Verification items for the finished model (mm, model axes). Face numbers are marked on the shaded views. A direction names the side the tool comes from. Coordinates: 2 decimals unless noted, no trailing zeros. Order: outer loops, then holes, each group sorted by start corner. A loop starts at its lowest first (then second) coordinate and runs counter-clockwise, first axis right, second up. Notation, with made-up numbers: M -9,11.5 L 38,11.5 A25 ccw 38,26.5 Z; hole C 15.25,52.25 d9. An arc over 180 degrees is marked long. Return JSON: item names as keys, results as strings.
```python
from build123d import *

# Parameters (mm, degrees)
SKETCH1_W                                            = 318
SKETCH1_H                                            = 160
BOSS_EXTRUDE1_DEPTH                                  = 25
SKETCH2_R                                            = 28.5
CUT_EXTRUDE1_DEPTH                                   = 180.738699228
CUT_EXTRUDE2_DEPTH                                   = 180.738699228
CUT_EXTRUDE2_DEPTH_BACK                              = 180.738699228
SKETCH4_R                                            = 9.55
CHAMFER1_SIZE                                        = 0.5
FILLET1_R                                            = 20
M8_CLEARANCE_HOLE1_D                                 = 9
M6X1_0_TAPPED_HOLE1_D                                = 5
SKETCH13_R                                           = 13.411040831
SKETCH13_R_2                                         = 14.724493856
BOSS_EXTRUDE3_DEPTH                                  = 8
CSK_FOR_5_16_FLAT_HEAD_SOCKET_CAP_SCREW1_D           = 8.4328
CSK_FOR_5_16_FLAT_HEAD_SOCKET_CAP_SCREW1_CSINK_D     = 18.4009792
CSK_FOR_5_16_FLAT_HEAD_SOCKET_CAP_SCREW1_CSINK_ANGLE = 82
BOSS_EXTRUDE4_DEPTH                                  = 6
CUT_EXTRUDE3_DEPTH                                   = 186.067555233
M6X1_0_TAPPED_HOLE2_D                                = 5
M6X1_0_TAPPED_HOLE2_DEPTH                            = 15
M6X1_0_TAPPED_HOLE2_TIP                              = 1.502151548
MIRROR2_COPY_1_DEPTH                                 = 186.067555233
CHAMFER4_SIZE                                        = 1


with BuildPart() as part:
    # Sketch1 → Boss-Extrude1 (new body)
    with BuildSketch(Plane(origin=(0, 0, 0), x_dir=(1, 0, 0), z_dir=(0, 1, 0))):
        Rectangle(SKETCH1_W, SKETCH1_H)
    extrude(amount=BOSS_EXTRUDE1_DEPTH)

    # Sketch2 → Cut-Extrude1 (cut, through all)
    with BuildSketch(Plane(origin=(0, 25, 0), x_dir=(1, 0, 0), z_dir=(0, 1, 0))):
        with Locations(Location((-114, 0, 0), (0, 0, 270))):
            Circle(SKETCH2_R)
        with Locations(Location((114, 0, 0), (0, 0, 270))):
            Circle(SKETCH2_R)
    extrude(amount=-CUT_EXTRUDE1_DEPTH, mode=Mode.SUBTRACT)

    # Sketch4 → Cut-Extrude2 (cut, two sides: drawn at the far end of the back side and taken through both)
    with BuildSketch(Plane(origin=(0, 25, 0), x_dir=(1, 0, 0), z_dir=(0, 1, 0)).offset(-CUT_EXTRUDE2_DEPTH_BACK)):
        with Locations(Location((-60, 0, 0), (0, 0, 270))):
            Circle(SKETCH4_R)
        with Locations(Location((60, 0, 0), (0, 0, 270))):
            Circle(SKETCH4_R)
    extrude(amount=CUT_EXTRUDE2_DEPTH + CUT_EXTRUDE2_DEPTH_BACK, mode=Mode.SUBTRACT)

    # Chamfer1
    chamfer1_edges = [part.edges().sort_by_distance(p)[0] for p in [
        (-114, 0, -28.5),
        (-114, 25, -28.5),
        (114, 0, -28.5),
        (114, 25, -28.5),
        (-60, 0, -9.55),
        (-60, 25, -9.55),
        (60, 0, -9.55),
        (60, 25, -9.55),
    ]]
    chamfer(chamfer1_edges, length=CHAMFER1_SIZE)

    # Fillet1
    fillet1_edges = [part.edges().sort_by_distance(p)[0] for p in [
        (159, 12.5, 80),
        (-159, 12.5, 80),
        (-159, 12.5, -80),
        (159, 12.5, -80),
    ]]
    fillet(fillet1_edges, radius=FILLET1_R)

    # M8 Clearance Hole1 (through all)
    with Locations(Plane.XZ):
        with Locations((-139, -60), (-139, 60), (139, -60), (139, 60)):
            Hole(M8_CLEARANCE_HOLE1_D / 2)

    # M6x1.0 Tapped Hole1 (through all)
    with Locations(Plane(origin=(0, 0, 0), x_dir=(-1, 0, 0), z_dir=(0, -1, 0))):
        with Locations((138.765, -24.765), (89.235, -24.765), (89.235, 24.765), (138.765, 24.765), (-89.235, -24.765), (-138.765, -24.765), (-89.235, 24.765), (-138.765, 24.765)):
            Hole(M6X1_0_TAPPED_HOLE1_D / 2)

    # Sketch13 → Boss-Extrude3 (add)
    with BuildSketch(Plane(origin=(0, 25, 0), x_dir=(1, 0, 0), z_dir=(0, 1, 0))):
        with Locations((60, 0)):
            Circle(SKETCH13_R)
        with Locations((-60, 0)):
            Circle(SKETCH13_R_2)
    extrude(amount=-BOSS_EXTRUDE3_DEPTH)

    # CSK for 5/16 Flat Head Socket Cap Screw1 (through all)
    with Locations(Plane(origin=(0, 25, 0), x_dir=(1, 0, 0), z_dir=(0, 1, 0))):
        with Locations((60, 0), (-60, 0)):
            CounterSinkHole(CSK_FOR_5_16_FLAT_HEAD_SOCKET_CAP_SCREW1_D / 2, CSK_FOR_5_16_FLAT_HEAD_SOCKET_CAP_SCREW1_CSINK_D / 2, counter_sink_angle=CSK_FOR_5_16_FLAT_HEAD_SOCKET_CAP_SCREW1_CSINK_ANGLE)

    # Sketch16 → Boss-Extrude4 (add)
    with BuildSketch(Plane.XZ.offset(-25)):
        with BuildLine():
            Line((163, -60), (163, 60))
            ThreePointArc((163, 60), (155.970562748, 76.970562748), (139, 84))
            Line((139, 84), (-139, 84))
            ThreePointArc((-139, 84), (-155.970562748, 76.970562748), (-163, 60))
            Line((-163, 60), (-163, -60))
            ThreePointArc((-163, -60), (-155.970562748, -76.970562748), (-139, -84))
            Line((-139, -84), (139, -84))
            ThreePointArc((139, -84), (155.970562748, -76.970562748), (163, -60))
        make_face()
        with BuildLine():
            Line((159, 60), (159, -60))
            ThreePointArc((159, -60), (153.142135624, -74.142135624), (139, -80))
            Line((139, -80), (-139, -80))
            ThreePointArc((-139, -80), (-153.142135624, -74.142135624), (-159, -60))
            Line((-159, -60), (-159, 60))
            ThreePointArc((-159, 60), (-153.142135624, 74.142135624), (-139, 80))
            Line((-139, 80), (139, 80))
            ThreePointArc((139, 80), (153.142135624, 74.142135624), (159, 60))
        make_face(mode=Mode.SUBTRACT)
    extrude(amount=BOSS_EXTRUDE4_DEPTH)

    # Sketch17 → Cut-Extrude3 (cut, through all)
    with BuildSketch(Plane.XZ):
        with BuildLine():
            Line((-60, -21.237304048), (-30, -21.237304048))
            ThreePointArc((-30, -21.237304048), (-16.218066161, -35.019237886), (-30, -48.801171725))
            Line((-30, -48.801171725), (-60, -48.801171725))
            ThreePointArc((-60, -48.801171725), (-73.781933839, -35.019237886), (-60, -21.237304048))
        make_face()
    cut_extrude3 = extrude(amount=-CUT_EXTRUDE3_DEPTH, mode=Mode.SUBTRACT)

    # M6x1.0 Tapped Hole2
    with Locations(Plane(origin=(0, 0, 0), x_dir=(-1, 0, 0), z_dir=(0, -1, 0))):
        with Locations((-75, 70), (-45, 70), (-105, 70), (-15, 70), (15, 70), (45, 70), (75, 70), (105, 70), (-105, -70), (-75, -70), (-45, -70), (-15, -70), (15, -70), (45, -70), (75, -70), (105, -70)):
            Hole(M6X1_0_TAPPED_HOLE2_D / 2, depth=M6X1_0_TAPPED_HOLE2_DEPTH)
            with Locations((0, 0, -(M6X1_0_TAPPED_HOLE2_DEPTH + M6X1_0_TAPPED_HOLE2_TIP / 2))):  # 118° drill point
                Cone(0, M6X1_0_TAPPED_HOLE2_D / 2, M6X1_0_TAPPED_HOLE2_TIP, mode=Mode.SUBTRACT)

    # Mirror1: Cut-Extrude3 across plane
    add(cut_extrude3.mirror(Plane(origin=(0, 0, 0), x_dir=(0, 0, 1), z_dir=(1, 0, 0))), mode=Mode.SUBTRACT)

    # Mirror2: Cut-Extrude3 across plane
    add(cut_extrude3.mirror(Plane.XY), mode=Mode.SUBTRACT)

    # Mirror2 copy 1 sketch → Mirror2 copy 1 (cut, through all)
    with BuildSketch(Plane(origin=(0, 0, 0), x_dir=(-1, 0, 0), z_dir=(0, -1, 0))):
        with BuildLine():
            Line((-60, -21.237304048), (-30, -21.237304048))
            ThreePointArc((-30, -21.237304048), (-16.218066161, -35.019237886), (-30, -48.801171725))
            Line((-30, -48.801171725), (-60, -48.801171725))
            ThreePointArc((-60, -48.801171725), (-73.781933839, -35.019237886), (-60, -21.237304048))
        make_face()
    extrude(amount=-MIRROR2_COPY_1_DEPTH, mode=Mode.SUBTRACT)

    # Chamfer4
    chamfer4_edges = [part.edges().sort_by_distance(p)[0] for p in [
        (-134.5, 0, 60),
        (-134.5, 25, 60),
        (-134.5, 0, -60),
        (-134.5, 25, -60),
        (155.970562748, 19, -76.970562748),
        (163, 19, 0),
        (155.970562748, 19, 76.970562748),
        (0, 19, 84),
        (-155.970562748, 19, 76.970562748),
        (-163, 19, 0),
        (-155.970562748, 19, -76.970562748),
        (0, 19, -84),
        (155.970562748, 25, -76.970562748),
        (163, 25, 0),
        (155.970562748, 25, 76.970562748),
        (0, 25, 84),
        (-155.970562748, 25, 76.970562748),
        (-163, 25, 0),
        (-155.970562748, 25, -76.970562748),
        (0, 25, -84),
        (-73.781933839, 25, -35.019237886),
        (-45, 25, -21.237304048),
        (-16.218066161, 25, -35.019237886),
        (-45, 25, -48.801171725),
        (-73.781933839, 0, -35.019237886),
        (-45, 0, -48.801171725),
        (-16.218066161, 0, -35.019237886),
        (-45, 0, -21.237304048),
        (73.781933839, 0, -35.019237886),
        (45, 0, -48.801171725),
        (16.218066161, 0, -35.019237886),
        (45, 0, -21.237304048),
        (73.781933839, 25, -35.019237886),
        (45, 25, -48.801171725),
        (16.218066161, 25, -35.019237886),
        (45, 25, -21.237304048),
        (73.781933839, 25, 35.019237886),
        (45, 25, 21.237304048),
        (16.218066161, 25, 35.019237886),
        (45, 25, 48.801171725),
        (73.781933839, 0, 35.019237886),
        (45, 0, 48.801171725),
        (16.218066161, 0, 35.019237886),
        (45, 0, 21.237304048),
        (-73.781933839, 0, 35.019237886),
        (-45, 0, 48.801171725),
        (-16.218066161, 0, 35.019237886),
        (-45, 0, 21.237304048),
        (-73.781933839, 25, 35.019237886),
        (-45, 25, 48.801171725),
        (-16.218066161, 25, 35.019237886),
        (-45, 25, 21.237304048),
        (159, 0, 0),
        (0, 0, 80),
        (-159, 0, 0),
        (0, 0, -80),
        (-153.142135624, 0, 74.142135624),
        (-153.142135624, 0, -74.142135624),
        (153.142135624, 0, -74.142135624),
        (153.142135624, 0, 74.142135624),
        (143.5, 0, 60),
        (143.5, 25, 60),
        (143.5, 0, -60),
        (143.5, 25, -60),
    ]]
    chamfer(chamfer4_edges, length=CHAMFER4_SIZE)


solid = part.part
```
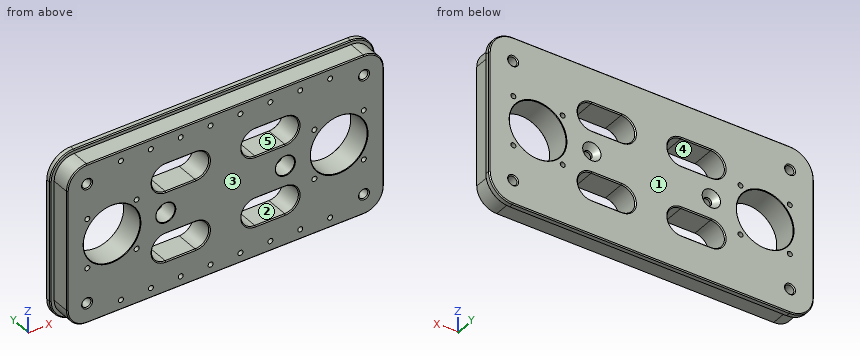
Q1. Cross-section at A-A, the plane x = -33. State how many separate pieces and enclosed holes the cut face has, and give its area (3 significant figures).
Values:
{"separate pieces": "3", "enclosed holes": "0", "area": "2,660 mm^2"}
Q2. Cross-section at B-B, the plane x = 114. Record the boundary of the cut face in (y, z), and give its area (3 significant figures).
Values:
{"outline": "M 0,-79 L 1,-80 L 19,-80 L 19,-83 L 20,-84 L 24,-84 L 25,-83 L 25,-29 L 24.5,-28.5 L 0.5,-28.5 L 0,-29 Z; M 0,29 L 0.5,28.5 L 24.5,28.5 L 25,29 L 25,83 L 24,84 L 20,84 L 19,83 L 19,80 L 1,80 L 0,79 Z", "area": "2,620 mm^2"}
Q3. Tool access check on the marked faces 1 and 2. Record the directions out of +Z, -Z, +X, -X, +Y, -Y that give a thin tool (end or side, any length) a straight path to the whole face; none if there is none.
Values:
{"face 1": "+Z, -Z, +X, -X, +Y", "face 2": "+Y, -Y"}
Q4. Material ranges on line 1 along Z through (x, y) = (-45, 8.75); line 2 along X through (y, z) = (3, -20.5); line 3 along Z through (x, y) = (105, 8), recorded low to high.
Values:
{"line 1": "-80 to -72.5, -67.5 to -48.8, -21.24 to 21.24, 48.8 to 67.5, 72.5 to 80", "line 2": "-159 to -133.8, -94.2 to 94.2, 133.8 to 159", "line 3": "-80 to -72.5, -67.5 to -27.04, 27.04 to 67.5, 72.5 to 80"}
Q5. Go/stop test with flat-tipped pins: pin 1 (4.5 mm diameter, centred on x = 138.765, z = -24.765, fed in from -Y); pin 2 (12 mm diameter, centred on x = -118.5, y = 10, fed in from -Z); pin 3 (12 mm diameter, centred on y = 10, z = -25, fed in from -X); pin 4 (12 mm diameter, centred on y = 10.5, z = 57.5, fed in from +X). Record where each tip stops, or that it passes through.
Values:
{"pin 1": "through", "pin 2": "z = -80", "pin 3": "x = -159", "pin 4": "x = 159"}
Q6. Draft check along Z on the marked faces 3, 4 and 5. Enter one of: pulls with the +Z half, pulls with the -Z half, needs draft (parallel to the pull), parting line crosses it, or undercut.
Values:
{"face 3": "needs draft", "face 4": "undercut", "face 5": "undercut"}
